Could you check a few things on this model? Use its own coordinates, in mm. Give positions to 0.01 mm unless a question says otherwise; leave off trailing zeros. Order: outer loops, then holes, each group sorted by start corner. A loop starts at its lowest first (then second) coordinate and runs counter-clockwise, first axis right, second up. Notation, with made-up numbers: M 22,21 L 33,21 A16 ccw 33,40 Z; hole C 22.25,50.25 d4. An arc over 180 degrees is marked long. Use a Markdown table: item, result. Add a question column.
Item 1: I'm going to push flat-ended pins straight in: pin 1 Ø0.6 at (x, y) = (83.5, 0.5) entering from -Z; pin 2 Ø1 at (x, y) = (-83.5, 0.5) entering from +Z; pin 3 Ø1 at (y, z) = (1, -64.5) entering from -X. Where does each tip first touch, or does it pass through?
Item 2: If we mould it in two halves opening along Y, with no side actions, what happens to faces 1 (the face through (-1, 0, -1)), 2 (the face through (-1, 2, -1))? For each: released by +Y, released by -Y, zero draft, split by the parting line, or undercut.
Item 3: If I drill on L1, parallel to X at y = 0.1, z = -53.5, over which ranges is the centre line in solid material (lowest first)? Write a range as from..to.
Item 4: Suppose I cut it at A-A on y = 0.35. Write out the boundary of the cut face in (x, z).
Item 5: Suppose I cut it at B-B on z = -21.5. Write out the boundary of the cut face in (x, y).
from build123d import *

# Parameters (mm, degrees)
SKETCH1_W           = 169.4
SKETCH1_H           = 150
BOSS_EXTRUDE1_DEPTH = 2
CUT_EXTRUDE1_DEPTH  = 2


with BuildPart() as part:
    # Sketch1 → Boss-Extrude1 (new body)
    with BuildSketch(Plane(origin=(0, 0, 0), x_dir=(1, 0, 0), z_dir=(0, 1, 0))):
        Rectangle(SKETCH1_W, SKETCH1_H)
    extrude(amount=BOSS_EXTRUDE1_DEPTH)

    # Sketch2 → Cut-Extrude1 (cut)
    with BuildSketch(Plane(origin=(0, 2, 0), x_dir=(1, 0, 0), z_dir=(0, 1, 0))):
        Polygon((82.5, -50), (82.5, -75), (87.923107592, -75), (87.923107592, 75), (82.5, 75), (82.5, 50), (84.7, 50), (84.7, 25), (82.5, 25), (82.5, -25), (84.7, -25), (84.7, -50), align=None)
        Polygon((-82.5, 50), (-82.5, 75), (-87.923107592, 75), (-87.923107592, -75), (-82.5, -75), (-82.5, -50), (-84.7, -50), (-84.7, -25), (-82.5, -25), (-82.5, 25), (-84.7, 25), (-84.7, 50), align=None)
    extrude(amount=-CUT_EXTRUDE1_DEPTH, mode=Mode.SUBTRACT)


solid = part.part
Findings below:
| question | item | result |
|---|---|---|
| 1 | pin 1 | stops at z = -50 |
| 1 | pin 2 | stops at z = 50 |
| 1 | pin 3 | stops at x = -82.5 |
| 2 | face 1 | released by -Y |
| 2 | face 2 | released by +Y |
| 3 | L1 | x = -82.5..82.5 |
| 4 | outline | M -84.7,-50 L -82.5,-50 L -82.5,-75 L 82.5,-75 L 82.5,-50 L 84.7,-50 L 84.7,-25 L 82.5,-25 L 82.5,25 L 84.7,25 L 84.7,50 L 82.5,50 L 82.5,75 L -82.5,75 L -82.5,50 L -84.7,50 L -84.7,25 L -82.5,25 L -82.5,-25 L -84.7,-25 Z |
| 5 | outline | M -82.5,0 L 82.5,0 L 82.5,2 L -82.5,2 Z |
